Could you check a few things on this model? Use its own coordinates, in mm. Face numbers are marked on the shaded views. Coordinates: 2 decimals unless noted, no trailing zeros. Write each loop counter-clockwise with the first axis right and the second up, starting at its lowest first coordinate (ties: lowest second). Pieces come first, ordered by that corner, then holes. Notation, with made-up numbers: M 53,85.25 L 99,85.25 A28 cw 99,113.25 Z; hole C 13,19.25 d4. An arc over 180 degrees is marked long. Write item = value, one per line.
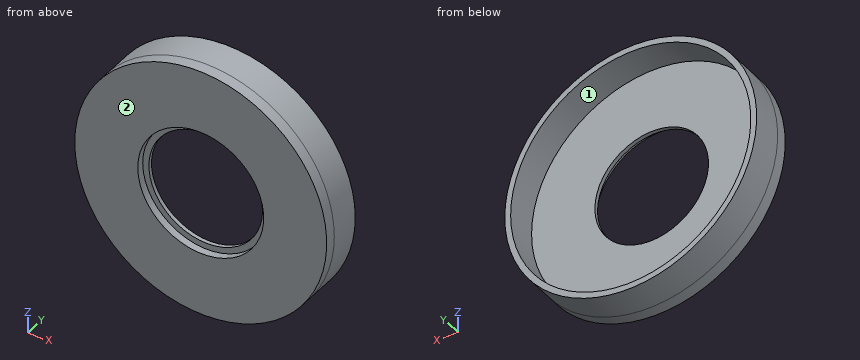
Autodesk Inventor part; units mm, degrees
ref_plane "YZ Plane" through (0, 0, 0) normal (1, 0, 0) x (0, 1, 0)
ref_plane "XZ Plane" through (0, 0, 0) normal (0, 1, 0) x (-1, 0, 0)
ref_plane "XY Plane" through (0, 0, 0) normal (0, 0, 1) x (1, 0, 0)
sketch "Sketch1" plane through (0, 0, 0) normal (0, 1, 0) x (-1, 0, 0)
  circle A0 centre (0, 0) radius 16.075
  circle A1 centre (0, 0) radius 32.15
  dimension "d0" = 32.15
  dimension "d1" = 64.3
extrude "Extrusion1" add sketch "Sketch1" along normal blind 1.9
sketch "Sketch2" plane through (0, 1.9, 0) normal (0, 1, 0) x (1, 0, 0)
  circle A0 centre (0, 0) radius 14.5
  circle A1 centre (0, 0) radius 32.15
  dimension "d4" = 29
extrude "Extrusion2" add sketch "Sketch2" along normal blind 1
sketch "Sketch3" plane through (0, 2.9, 0) normal (0, 1, 0) x (1, 0, 0)
  circle A0 centre (0, 0) radius 30.65
  circle A1 centre (0, 0) radius 32.15
  dimension "d7" = 61.3
  dimension "d10" = 64.3
extrude "Extrusion3" add sketch "Sketch3" along normal blind 8
properties part number "Widefield_LightShield_LowerRing"
Item 1: If we mould it in two halves opening along X, with no side actions, what happens to the marked faces 1 and 2? For each: pulls with the +X half, pulls with the -X half, needs draft (parallel to the pull), parting line crosses it, or undercut.
Numbers:
face_1 = undercut
face_2 = needs draft
Item 2: Imagine slicing it at B-B (z = -20.5). Write out the boundary of the cut face in (x, y).
Numbers:
outline = M -24.77,0 L 24.77,0 L 24.77,10.9 L 22.79,10.9 L 22.79,2.9 L -22.79,2.9 L -22.79,10.9 L -24.77,10.9 Z
Item 3: If I drill on line 1 along Z through (x, y) = (0, 8); line 2 along Z through (x, y) = (0, 2.2), over which ranges is the centre line in solid material (lowest first)?
Numbers:
line_1 = -32.15 to -30.65, 30.65 to 32.15
line_2 = -32.15 to -14.5, 14.5 to 32.15
Item 4: Imagine slicing it at C-C (y = 9). Write out the boundary of the cut face in (x, z).
Numbers:
outline = C 0,0 d64.3; hole C 0,0 d61.3
Item 5: I'm going to push flat-ended pins straight in: P1, Ø4, axis at x = 25, y = 4.5, coming from the -Z side; P2, Ø3, axis at x = 20.5, z = 18.5, coming from the +Y side; P3, Ø1, axis at x = 12.5, y = 4, coming from the +Z side. Where does each tip first touch, or does it pass through?
Numbers:
P1 = -22.46
P2 = 2.9
P3 = 29.83
